Design review of the part built by this model. Coordinates are the model's own, in mm. A direction names the side the tool comes from. Coordinates: 2 decimals unless noted, no trailing zeros. Write each loop counter-clockwise with the first axis right and the second up, starting at its lowest first coordinate (ties: lowest second). Pieces come first, ordered by that corner, then holes. Notation, with made-up numbers: (40.5, -23) -> (45.5, -23) arc R24 cw to (45.5, 1) -> close; hole circle Ø3 at (25.25, 60). An arc over 180 degrees is marked (long way). Answer in a Markdown table with one row per item. Add a question column.
Item 1: Take a section at A-A, the plane y = -57. Write out the cut boundary in (x, z), and give its area (3 significant figures).
Item 2: Take a section at B-B, the plane z = 13. Give the number of separate pieces and of enclosed holes in the cut face, and give its area (3 significant figures).
Item 3: Clearance check with flat-ended pins moving along their axes: P1, Ø10, axis at x = -1482.27, y = 27.41, coming from the -Z side; P2, Ø1.1, axis at x = -1452.5, y = -159, coming from the +Z side; P3, Ø1.1, axis at x = -1465, y = -159, coming from the -Z side; P4, Ø12, axis at y = -120.5, z = 5, coming from the -X side. State where each tip first meets the part, or that it passes through.
Item 4: To check wall thickness, follow line 1 (X direction, y = 27.5, z = 25.5); line 2 (Y direction, x = -1419, z = 17); line 3 (Y direction, x = -1436.5, z = 15.5). State the ranges of each line that lie inside material, in increasing order.
Item 5: Draft analysis for pull direction Y (two halves, no side actions). For faces 4 (the face through (-1445, -160, 25)), 5 (the face through (-1424.723, -15.56, 18.944)), 6 (the face through (-1460.21, -162.23, 18.57)), state which applies: released by +Y, released by -Y, zero draft, split by the parting line, or undercut.
Item 6: For faces 1 (the face through (-1444.044, 27.69, 30.07)), 2 (the face through (-1422, 25, 23)), 3 (the face through (-1434, -150, 25)), list the 3-axis set-ups (+Z, -Z, +X, -X, +Y, -Y) from which the entire face can be reached by the end or side of a thin tool; tool diameter is ignored.
from build123d import *

# Parameters (mm, degrees)
ESTRUSIONE_ESTRUSIONE2_DEPTH      = 1
ESTRUSIONE_ESTRUSIONE2_2_DEPTH    = 1
ESTRUSIONE_ESTRUSIONE3_DEPTH      = 15
SCHIZZO4_W                        = 100
SCHIZZO4_H                        = 79
ESTRUSIONE_ESTRUSIONE4_DEPTH      = 20
TAGLIO_ESTRUSIONE2_DEPTH          = 36
RACCORDO1_R                       = 1
ESTRUSIONE_ESTRUSIONE5_DEPTH      = 20
ESTRUSIONE_ESTRUSIONE6_DEPTH      = 30
SCHIZZO11_W                       = 20
SCHIZZO11_H                       = 5
ESTRUSIONE_ESTRUSIONE7_DEPTH      = 17.5
ESTRUSIONE_ESTRUSIONE7_DEPTH_BACK = 47.5
TAGLIO_ESTRUSIONE5_REACH          = 201.338
SCHIZZO13_R                       = 2.5
SCHIZZO14_R                       = 6.3235
SCHIZZO14_R_2                     = 3.3235
TAGLIO_ESTRUSIONE6_DEPTH          = 10
TAGLIO_ESTRUSIONE7_DEPTH          = 20
SCHIZZO7_R                        = 6
TAGLIO_ESTRUSIONE4_DEPTH          = 8


with BuildPart() as part:
    # Schizzo1 → Estrusione-Estrusione2 (new body)
    with BuildSketch(Plane.XY):
        with BuildLine():
            ThreePointArc((-1482, 0), (-1485, 3), (-1488, 0))
            ThreePointArc((-1488, 0), (-1485, -3), (-1482, 0))
        make_face()
    extrude(amount=-ESTRUSIONE_ESTRUSIONE2_DEPTH)



with BuildPart() as body_2:
    # Schizzo1 → Estrusione-Estrusione2 2 (new body)
    with BuildSketch(Plane.XY):
        with BuildLine():
            ThreePointArc((-1475.75, 0), (-1460, -15.75), (-1444.25, 0))
            ThreePointArc((-1444.25, 0), (-1460, 15.75), (-1475.75, 0))
        make_face()
    extrude(amount=-ESTRUSIONE_ESTRUSIONE2_2_DEPTH)


with BuildPart() as part_1:
    add(part.part)

    add(body_2.part)  # Estrusione-Estrusione3 merges body 2
    # Schizzo2 → Estrusione-Estrusione3 (add)
    with BuildSketch(Plane.XY):
        with BuildLine():
            Line((-1423, 14.138214937), (-1423, 18.085801585))
            add(Edge.make_bspline(
                [(-1423, 18.085801585), (-1424.815922694, 23.27497966), (-1427.541323769, 28.145982802), (-1431.102851615, 32.485450033), (-1439.594271418, 39.731973592), (-1450.044163239, 43.658327797), (-1455.564993498, 44.676158034), (-1466.7280127, 44.734359641), (-1477.245308948, 40.992328412), (-1482.120117986, 38.208118184), (-1490.68666297, 31.050559385), (-1496.308059, 21.406065909), (-1498.236323874, 16.133743979), (-1500.163676126, 5.138214937), (-1498.236323874, -5.857314104), (-1496.308059, -11.129636034), (-1490.68666297, -20.774129511), (-1482.120117986, -27.931688309), (-1477.245308948, -30.715898537), (-1466.7280127, -34.457929766), (-1455.564993498, -34.399728159), (-1450.044163239, -33.381897922), (-1439.594271418, -29.455543717), (-1431.102851615, -22.209020158), (-1427.541323769, -17.869552928), (-1424.815922694, -12.998549785), (-1422.999999932, -7.809371515)],
                knots=[-1.234179621, -1.234179621, -1.234179621, -1.234179621, -1.234179621, -1.234179621, -0.532935634, -0.532935634, -0.532935634, 0.168308353, 0.168308353, 0.168308353, 0.86955234, 0.86955234, 0.86955234, 1.570796327, 1.570796327, 1.570796327, 2.272040314, 2.272040314, 2.272040314, 2.973284301, 2.973284301, 2.973284301, 3.674528288, 3.674528288, 3.674528288, 4.375772275, 4.375772275, 4.375772275, 4.375772275, 4.375772275, 4.375772275], degree=5))
            Line((-1422.999999932, -7.809371515), (-1423, -3.861785063))
            Line((-1423, -3.861785063), (-1421.847149517, -3.861785063))
            ThreePointArc((-1421.847149517, -3.861785063), (-1420.8, 5.138214937), (-1421.847149517, 14.138214937))
            Line((-1421.847149517, 14.138214937), (-1423, 14.138214937))
        make_face()
        with BuildLine():
            ThreePointArc((-1437.726136393, 30.735578545), (-1441.049636393, 27.412078545), (-1437.726136393, 24.088578545))
            ThreePointArc((-1437.726136393, 24.088578545), (-1434.402636393, 27.412078545), (-1437.726136393, 30.735578545))
        make_face(mode=Mode.SUBTRACT)
        with BuildLine():
            ThreePointArc((-1437.726136393, -13.81214867), (-1441.049636393, -17.13564867), (-1437.726136393, -20.45914867))
            ThreePointArc((-1437.726136393, -20.45914867), (-1434.402636393, -17.13564867), (-1437.726136393, -13.81214867))
        make_face(mode=Mode.SUBTRACT)
        with BuildLine():
            ThreePointArc((-1482.273863607, -13.81214867), (-1485.597363607, -17.13564867), (-1482.273863607, -20.45914867))
            ThreePointArc((-1482.273863607, -20.45914867), (-1478.950363607, -17.13564867), (-1482.273863607, -13.81214867))
        make_face(mode=Mode.SUBTRACT)
        with BuildLine():
            ThreePointArc((-1482.273863607, 30.735578545), (-1485.597363607, 27.412078545), (-1482.273863607, 24.088578545))
            ThreePointArc((-1482.273863607, 24.088578545), (-1478.950363607, 27.412078545), (-1482.273863607, 30.735578545))
        make_face(mode=Mode.SUBTRACT)
    extrude(amount=ESTRUSIONE_ESTRUSIONE3_DEPTH)

    # Schizzo4 → Estrusione-Estrusione4 (add)
    with BuildSketch(Plane.XY.offset(15)):
        with Locations((-1460, 4.838223987)):
            Rectangle(SCHIZZO4_W, SCHIZZO4_H)
    extrude(amount=ESTRUSIONE_ESTRUSIONE4_DEPTH)

    # Schizzo5 → Taglio-Estrusione2 (cut)
    with BuildSketch(Plane(origin=(0, 0, -1), x_dir=(-1, 0, 0), z_dir=(0, 0, -1))):
        with BuildLine():
            ThreePointArc((1437.726136393, -13.81214867), (1434.402636393, -17.13564867), (1437.726136393, -20.45914867))
            ThreePointArc((1437.726136393, -20.45914867), (1441.049636393, -17.13564867), (1437.726136393, -13.81214867))
        make_face()
        with BuildLine():
            ThreePointArc((1437.726136393, 24.088578545), (1441.049636393, 27.412078545), (1437.726136393, 30.735578545))
            ThreePointArc((1437.726136393, 30.735578545), (1434.402636393, 27.412078545), (1437.726136393, 24.088578545))
        make_face()
        with BuildLine():
            ThreePointArc((1482.273863607, 24.088578545), (1485.597363607, 27.412078545), (1482.273863607, 30.735578545))
            ThreePointArc((1482.273863607, 30.735578545), (1478.950363607, 27.412078545), (1482.273863607, 24.088578545))
        make_face()
        with BuildLine():
            ThreePointArc((1482.273863607, -20.45914867), (1485.597363607, -17.13564867), (1482.273863607, -13.81214867))
            ThreePointArc((1482.273863607, -13.81214867), (1478.950363607, -17.13564867), (1482.273863607, -20.45914867))
        make_face()
    extrude(amount=-TAGLIO_ESTRUSIONE2_DEPTH, mode=Mode.SUBTRACT)

    # Raccordo1
    raccordo1_edges = [part_1.edges().sort_by_distance(p)[0] for p in [
        (-1510, -34.661776013, 25),
        (-1510, 44.338223987, 25),
        (-1410, -34.661776013, 25),
        (-1410, 44.338223987, 25),
    ]]
    fillet(raccordo1_edges, radius=RACCORDO1_R)

    # Schizzo8 → Estrusione-Estrusione5 (add)
    with BuildSketch(Plane.XY.offset(35)):
        Polygon((-1460, -34.661776013), (-1475, -34.661776013), (-1475, -155), (-1465.76, -155), (-1445, -155), (-1445, -34.661776013), align=None)
    extrude(amount=-ESTRUSIONE_ESTRUSIONE5_DEPTH)

    # Schizzo10 → Estrusione-Estrusione6 (add)
    with BuildSketch(Plane.ZY.offset(1475)):
        Polygon((20.7, -155), (20.7, -156.76), (16.7, -156.76), (16.7, -160.36), (20.483021279, -164.143021279), (29.516978721, -164.143021279), (33.3, -160.36), (33.3, -156.76), (29.3, -156.76), (29.3, -155), align=None)
    extrude(amount=-ESTRUSIONE_ESTRUSIONE6_DEPTH)

    # Schizzo11 → Estrusione-Estrusione7 (add, two sides)
    with BuildSketch(Plane(origin=(-1445, 0, 0), x_dir=(0, 0, -1), z_dir=(1, 0, 0))) as estrusione_estrusione7_sk:
        with Locations((-25, -152.5)):
            Rectangle(SCHIZZO11_W, SCHIZZO11_H)
    extrude(amount=ESTRUSIONE_ESTRUSIONE7_DEPTH)
    extrude(estrusione_estrusione7_sk.sketch, amount=-ESTRUSIONE_ESTRUSIONE7_DEPTH_BACK)

    # Schizzo13 → Taglio-Estrusione5 (cut, up to next)
    with BuildSketch(Plane.XZ.offset(155), mode=Mode.PRIVATE) as taglio_estrusione5_sk1:
        with Locations((-1437.15, 25)):
            Circle(SCHIZZO13_R)
    taglio_estrusione5_tool1 = extrude(taglio_estrusione5_sk1.sketch, amount=-TAGLIO_ESTRUSIONE5_REACH, mode=Mode.PRIVATE) & part_1.part
    add(taglio_estrusione5_tool1.solids().sort_by_distance((-1437.15, -155, 25))[0], mode=Mode.SUBTRACT)
    # Schizzo13 → Taglio-Estrusione5 (cut, up to next)
    with BuildSketch(Plane.XZ.offset(155), mode=Mode.PRIVATE) as taglio_estrusione5_sk2:
        with Locations((-1482.85, 25)):
            Circle(SCHIZZO13_R)
    taglio_estrusione5_tool2 = extrude(taglio_estrusione5_sk2.sketch, amount=-TAGLIO_ESTRUSIONE5_REACH, mode=Mode.PRIVATE) & part_1.part
    add(taglio_estrusione5_tool2.solids().sort_by_distance((-1482.85, -155, 25))[0], mode=Mode.SUBTRACT)

    # Schizzo14 → Taglio-Estrusione6 (cut)
    with BuildSketch(Plane.XY.offset(35)):
        with Locations((-1482.273863607, 27.412078545)):
            Circle(SCHIZZO14_R)
        with Locations((-1482.273863607, 27.412078545)):
            Circle(SCHIZZO14_R_2, mode=Mode.SUBTRACT)
        with Locations((-1482.273863607, -17.13564867)):
            Circle(SCHIZZO14_R)
        with Locations((-1482.273863607, -17.13564867)):
            Circle(SCHIZZO14_R_2, mode=Mode.SUBTRACT)
        with Locations((-1437.726136393, -17.13564867)):
            Circle(SCHIZZO14_R)
        with Locations((-1437.726136393, -17.13564867)):
            Circle(SCHIZZO14_R_2, mode=Mode.SUBTRACT)
        with Locations((-1437.726136393, 27.412078545)):
            Circle(SCHIZZO14_R)
        with Locations((-1437.726136393, 27.412078545)):
            Circle(SCHIZZO14_R_2, mode=Mode.SUBTRACT)
    extrude(amount=-TAGLIO_ESTRUSIONE6_DEPTH, mode=Mode.SUBTRACT)

    # Schizzo15 → Taglio-Estrusione7 (cut)
    with BuildSketch(Plane.XY.offset(35)):
        with BuildLine():
            ThreePointArc((-1419, 24.238214937), (-1415.6, 27.638214937), (-1419, 31.038214937))
            ThreePointArc((-1419, 31.038214937), (-1422.4, 27.638214937), (-1419, 24.238214937))
        make_face()
        with BuildLine():
            ThreePointArc((-1419, -13.961785063), (-1422.4, -17.361785063), (-1419, -20.761785063))
            ThreePointArc((-1419, -20.761785063), (-1415.6, -17.361785063), (-1419, -13.961785063))
        make_face()
        with BuildLine():
            ThreePointArc((-1501, -13.961785063), (-1504.4, -17.361785063), (-1501, -20.761785063))
            ThreePointArc((-1501, -20.761785063), (-1497.6, -17.361785063), (-1501, -13.961785063))
        make_face()
        with BuildLine():
            ThreePointArc((-1501, 31.038214937), (-1504.4, 27.638214937), (-1501, 24.238214937))
            ThreePointArc((-1501, 24.238214937), (-1497.6, 27.638214937), (-1501, 31.038214937))
        make_face()
    extrude(amount=-TAGLIO_ESTRUSIONE7_DEPTH, mode=Mode.SUBTRACT)

    # Schizzo7 → Taglio-Estrusione4 (cut)
    with BuildSketch(Plane(origin=(0, 0, 15), x_dir=(-1, 0, 0), z_dir=(0, 0, -1))):
        with Locations((1419, 27.638214937)):
            Circle(SCHIZZO7_R)
        with Locations((1501, -17.361785063)):
            Circle(SCHIZZO7_R)
        with Locations((1501, 27.638214937)):
            Circle(SCHIZZO7_R)
        with Locations((1419, -17.361785063)):
            Circle(SCHIZZO7_R)
    extrude(amount=-TAGLIO_ESTRUSIONE4_DEPTH, mode=Mode.SUBTRACT)


solid = part_1.part
Answers:
| question | item | result |
|---|---|---|
| 1 | outline | (-1475, 15) -> (-1445, 15) -> (-1445, 35) -> (-1475, 35) -> close |
| 1 | area | 600 mm^2 |
| 2 | separate pieces | 1 |
| 2 | enclosed holes | 4 |
| 2 | area | 4,680 mm^2 |
| 3 | P1 | stops at z = 0 |
| 3 | P2 | stops at z = 33.3 |
| 3 | P3 | stops at z = 16.7 |
| 3 | P4 | passes through |
| 4 | line 1 | x = -1510 to -1504.4, -1497.6 to -1488.6, -1475.95 to -1444.05, -1431.4 to -1422.4, -1415.6 to -1410 |
| 4 | line 2 | y = -34.66 to -23.36, -11.36 to 21.64, 33.64 to 44.34 |
| 4 | line 3 | y = -155 to -150, -34.66 to -20.22, -14.05 to 24.32, 30.5 to 44.34 |
| 5 | face 4 | zero draft |
| 5 | face 5 | undercut |
| 5 | face 6 | released by -Y |
| 6 | face 1 | +Z |
| 6 | face 2 | -Z |
| 6 | face 3 | +Z, -Z, +X |
